For this review, use the dimensioned drawing (mm, ordinates from the lowest corner) and the shaded views. A direction names the side the tool comes from. Round coordinates to 2 decimals unless told otherwise and drop trailing zeros. Loops run counter-clockwise (first coordinate to the right, second up) from the corner with the lowest first, then second, coordinate; pieces in that order, holes last. Notation, with made-up numbers: (9.5, 65.25) - (54.5, 65.25) arc R28 cw to (54.5, 88.25) - close; hole circle Ø4 at (68.25, -11). An arc over 180 degrees is marked (long way). Answer as CSV lines item,"result". Start each with the question number.
(1) Consider section A-A (z = 36). Give the boundary of the cut face in (x, y), and give its area (3 significant figures).
(2) Consider section B-B (y = 36). Give the boundary of the cut face in (x, z).
(3) Consider section C-C (x = 68.5). Give the boundary of the cut face in (y, z), and give its area (3 significant figures).
(4) For P1, Ø6, axis at x = 15, z = 58, coming from the -Y side; P2, Ø4, axis at y = 8, z = 10, coming from the -X side; P3, Ø6, axis at x = 61.5, y = 64.5, coming from the -Z side; P4, Ø1.5, axis at x = 112, y = 44.5, coming from the -Z side, all flat-tipped, find the tip position at first contact; note any pin that passes through.
(5) For the marked faces 1, 2 and 3, list the 3-axis set-ups (+Z, -Z, +X, -X, +Y, -Y) from which the entire face can be reached by the end or side of a thin tool; tool diameter is ignored.
(6) Wall thickness on L1, parallel to Y at x = 119.5, z = 36; L2, parallel to X at y = 36, z = 8; L3, parallel to Z at x = 91, y = 14: over which ranges is each line inside the solid? List them lowest first.
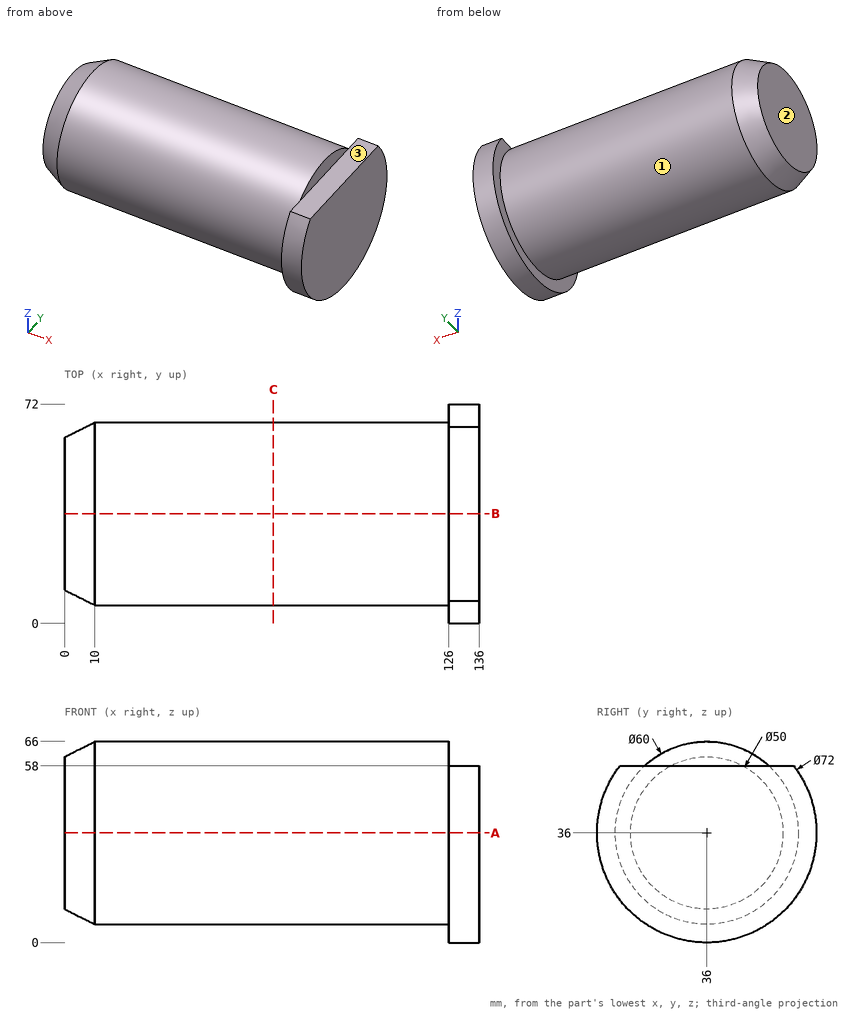
Determined:
1,outline,"(0, 11) - (10, 6) - (126, 6) - (126, 0) - (136, 0) - (136, 72) - (126, 72) - (126, 66) - (10, 66) - (0, 61) - close"
1,area,"8,230 mm^2"
2,outline,"(0, 11) - (10, 6) - (126, 6) - (126, 0) - (136, 0) - (136, 58) - (126, 58) - (126, 66) - (10, 66) - (0, 61) - close"
3,outline,"circle Ø60 at (36, 36)"
3,area,"2,830 mm^2"
4,P1,"stops at y = 12.78"
4,P2,"passes through"
4,P3,"stops at z = 20.2"
4,P4,"stops at z = 7.02"
5,face 1,"-X"
5,face 2,"+Z, -Z, -X, +Y, -Y"
5,face 3,"+Z, +X, +Y, -Y"
6,L1,"y = 6 to 66"
6,L2,"x = 6 to 136"
6,L3,"z = 15.6 to 56.4"
